Autodesk Inventor part; units mm, degrees
ref_plane "YZ Plane" through (0, 0, 0) normal (1, 0, 0) x (0, 1, 0)
ref_plane "XZ Plane" through (0, 0, 0) normal (0, 1, 0) x (-1, 0, 0)
ref_plane "XY Plane" through (0, 0, 0) normal (0, 0, 1) x (1, 0, 0)
sketch "Skizze1" plane through (0, 0, 0) normal (0, 0, 1) x (1, 0, 0)
  line L0 (-6.3, 6.3) -> (6.3, 6.3)
  line L1 (6.3, 6.3) -> (6.3, -6.3)
  line L2 (6.3, -6.3) -> (-6.3, -6.3)
  line L3 (-6.3, -6.3) -> (-6.3, 6.3)
  circle A0 centre (0, 0) radius 6.3
  circle A1 centre (0, 0) radius 5.3
  circle A2 centre (0, 0) radius 5.3
  circle A3 centre (0, 0) radius 6.3
  point P0 (0, -6.3)
  point P1 (-6.3, 0)
  dimension "d0" = 12.6
  dimension "d1" = 12.6
  dimension "d23" = 10.6
extrude "Extrusion2" add sketch "Skizze1" along normal blind 3
sketch "Skizze2" plane through (0, 0, 3) normal (0, 0, 1) x (1, 0, 0)
  circle A0 centre (0, 0) radius 5.3
  circle A1 centre (0, 0) radius 6.3
  dimension "d7" = 12.6
extrude "Extrusion3" add sketch "Skizze2" along normal blind 8
sketch "Skizze3" plane through (0, 0, 0) normal (0, 0, -1) x (-1, 0, 0)
  circle A0 centre (0, 0) radius 5.3
  circle A1 centre (0, 0) radius 5.3
  circle A2 centre (0, 0) radius 6.25
  dimension "d10" = 12.5
extrude "Extrusion4" add sketch "Skizze3" along normal blind 24
sketch "Skizze4" plane through (0, 0, -24) normal (0, 0, -1) x (-1, 0, 0)
  circle A0 centre (0, 0) radius 6.25
  circle A1 centre (0, 0) radius 5.3
  line L0 (-6.35, -6.35) -> (6.25, -6.35)
  line L1 (6.25, -6.35) -> (6.25, 6.25)
  line L2 (6.25, 6.25) -> (-6.35, 6.25)
  line L3 (-6.35, 6.25) -> (-6.35, -6.35)
  dimension "d25" = 10.6
  dimension "d26" = 12.5
  dimension "d29" = 12.6
  dimension "d30" = 12.6
sketch "Skizze5" plane through (6.3, 6.3, 3) normal (0, 1, 0) x (1, 0, 0)
  point P0 (-6.75, 1.5)
hole "Hole1" at (-0.45, 6.3, 1.5) direction (0, -1, 0) diameter 2 depth 8 tip angle 118
extrude "Extrusion6" add sketch "Skizze4" against normal blind 2.5 contours L1 L0 L3 L2 A0 | A0 L2 L1
properties part number "Sicherungshalter"
Geometry check sheet. Reference: the model listing, model coordinates, mm. A direction names the side the tool comes from. Round coordinates to 2 decimals unless told otherwise and drop trailing zeros. Order: outer loops, then holes, each group sorted by start corner. A loop starts at its lowest first (then second) coordinate and runs counter-clockwise, first axis right, second up. Notation, with made-up numbers: (85.25, 21.25) - (120.25, 21.25) arc R15 cw to (120.25, 31.25) - close; hole circle Ø6 at (-33, 63). An arc over 180 degrees is marked (long way). Use a Markdown table: item, result. Add a question column.
1) Section check D-D (x = -0.45). Count the separate pieces of the cut face and the enclosed holes in it, then the cut area to 3 significant figures.
2) Mould release check, pull along Z, two halves, no side actions. Record for faces 1 (the flat face through (6, 0, -24)), 2 (the flat face through (0, -6.35, -23)), 3 (the flat face through (-5, 5, -21.5)): released by +Z, released by -Z, zero draft, split by the parting line, or undercut.
3) Set-up check for faces 4 (the flat face through (0, -6.3, 1)), 5 (the flat face through (5, 5, 3)), 6 (the flat face through (6.3, 0, 1)): record each of +Z, -Z, +X, -X, +Y, -Y from which the full face is reachable in a straight line by a thin tool's end or side.
4) Section check A-A (x = 2.5). Record the cut outline in (y, z), then the cut area to 3 significant figures.
5) Gauge pin test, flat ends, axial feed: P1, Ø0.9, axis at y = 0.5, z = 2, coming from the +X side; P2, Ø0.8, axis at y = -1, z = -22.5, coming from the -X side; P3, Ø1, axis at x = -5, z = -9, coming from the -Y side; P4, Ø6.5, axis at x = 0, y = 0, coming from the +Z side. Record the tip position at first contact, or that the pin passes through.
6) Thickness scan on line 1 along Y through (x, z) = (0, 7.25); line 2 along X through (y, z) = (5.7, 1.5). Record the ranges inside material, lowest first.
7) Section check B-B (y = 3.25). Record the cut outline in (x, z).
8) Section check C-C (z = -16). Record the cut outline in (x, y), then the cut area to 3 significant figures.
Established:
| question | item | result |
|---|---|---|
| 1 | separate pieces | 3 |
| 1 | enclosed holes | 0 |
| 1 | area | 66.2 mm2 |
| 2 | face 1 | released by -Z |
| 2 | face 2 | zero draft |
| 2 | face 3 | undercut |
| 3 | face 4 | +Z, +X, -X, -Y |
| 3 | face 5 | +Z, +X, +Y |
| 3 | face 6 | +Z, +X, +Y, -Y |
| 4 | outline | (-6.35, -24) - (-4.67, -24) - (-4.67, 11) - (-5.78, 11) - (-5.78, 3) - (-6.3, 3) - (-6.3, 0) - (-5.73, 0) - (-5.73, -21.5) - (-6.35, -21.5) - close; (4.67, -24) - (6.25, -24) - (6.25, -21.5) - (5.73, -21.5) - (5.73, 0) - (6.3, 0) - (6.3, 3) - (5.78, 3) - (5.78, 11) - (4.67, 11) - close |
| 4 | area | 81.0 mm2 |
| 5 | P1 | x = 6.3 |
| 5 | P2 | x = -6.25 |
| 5 | P3 | y = -4.34 |
| 5 | P4 | through |
| 6 | line 1 | -6.3 to -5.3, 5.3 to 6.3 |
| 6 | line 2 | -6.3 to -1.45, 0.55 to 6.3 |
| 7 | outline | (-6.3, 0) - (-5.34, 0) - (-5.34, -21.5) - (-6.25, -21.5) - (-6.25, -24) - (-4.19, -24) - (-4.19, 11) - (-5.4, 11) - (-5.4, 3) - (-6.3, 3) - close; (4.19, -24) - (6.35, -24) - (6.35, -21.5) - (5.34, -21.5) - (5.34, 0) - (6.3, 0) - (6.3, 3) - (5.4, 3) - (5.4, 11) - (4.19, 11) - close |
| 8 | outline | circle Ø12.5 at (0, 0); hole circle Ø10.6 at (0, 0) |
| 8 | area | 34.5 mm2 |
